Could you check a few things on this drawing? It's one solid part, dimensions in mm from its lowest x, y, z. Round coordinates to 2 decimals unless told otherwise and drop trailing zeros. Write each loop counter-clockwise with the first axis right and the second up, starting at its lowest first coordinate (ties: lowest second). Pieces come first, ordered by that corner, then holes. Notation, with made-up numbers: M 22,18.5 L 57,18.5 A27 ccw 57,50.5 Z; hole C 75.5,41 d4. An arc over 180 degrees is marked long. One line per question, with ' | ' between items. Start each with the question number.
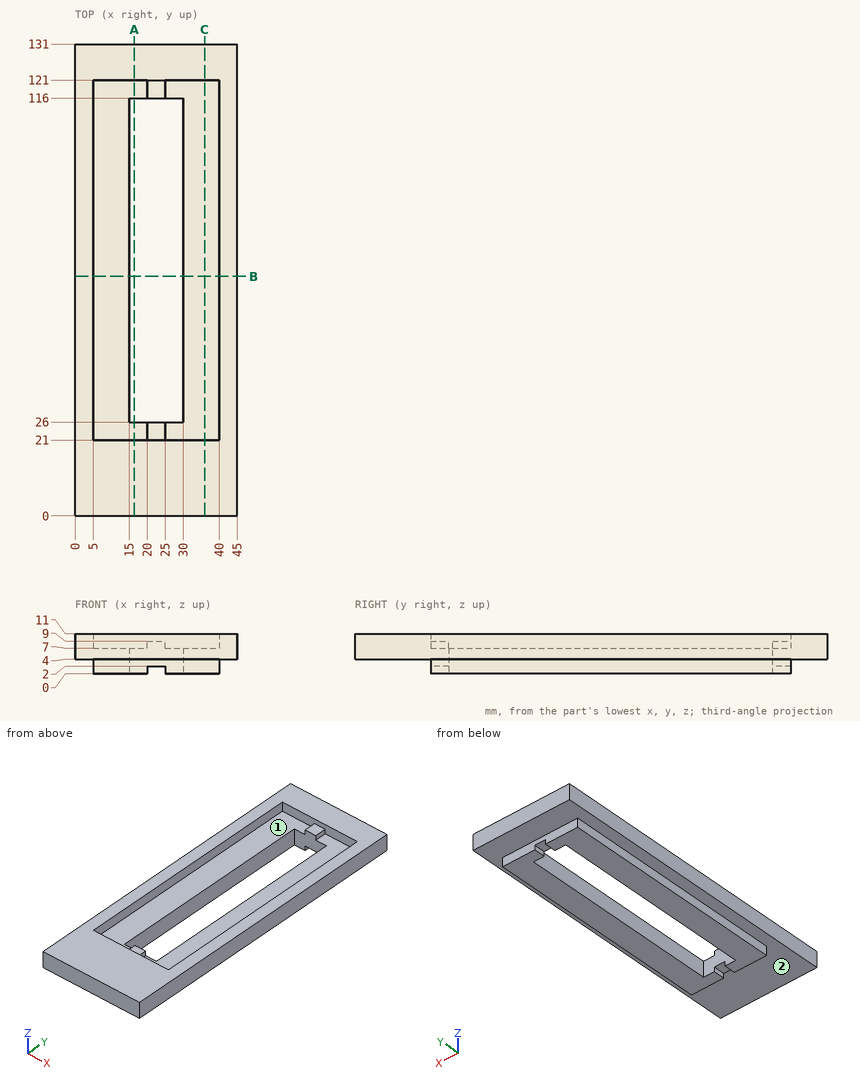
1. Suppose I cut it at C-C (x = 36). Write out the boundary of the cut face in (y, z), and give its area (3 significant figures).
2. I need wall thicknesses on line 1 along Y through (x, z) = (19.5, 1.75); line 2 along X through (y, z) = (95.5, 9.25); line 3 along X through (y, z) = (62, 3.25). Which ranges of each line are inside material? Lowest first, please. Write a range as from..to.
3. Suppose I cut it at A-A (x = 16.5). Write out the boundary of the cut face in (y, z).
4. Suppose I cut it at B-B (y = 66.5). Write out the boundary of the cut face in (x, z), and give its area (3 significant figures).
5. I'm going to push flat-ended pins straight in: P1, Ø7.5, axis at x = 11.5, y = 54, coming from the +Z side; P2, Ø0.6, axis at y = 23, z = 1, coming from the +X side; P3, Ø1, axis at y = 23.5, z = 0.5, coming from the -X side. Where does each tip first touch, or does it pass through?
6. If we mould it in two halves opening along Y, with no side actions, what happens to the marked faces 1 and 2? For each: released by +Y, released by -Y, zero draft, split by the parting line, or undercut.
Computed:
1) outline: M 0,4 L 21,4 L 21,0 L 121,0 L 121,4 L 131,4 L 131,11 L 121,11 L 121,7 L 21,7 L 21,11 L 0,11 Z | area: 917 mm²
2) line 1: y = 21..26, 116..121 | line 2: x = 0..5, 40..45 | line 3: x = 5..15, 30..40
3) outline: M 0,4 L 21,4 L 21,0 L 26,0 L 26,7 L 21,7 L 21,11 L 0,11 Z; M 116,0 L 121,0 L 121,4 L 131,4 L 131,11 L 121,11 L 121,7 L 116,7 Z
4) outline: M 0,4 L 5,4 L 5,0 L 15,0 L 15,7 L 5,7 L 5,11 L 0,11 Z; M 30,0 L 40,0 L 40,4 L 45,4 L 45,11 L 40,11 L 40,7 L 30,7 Z | area: 210 mm²
5) P1: stops at z = 7 | P2: stops at x = 40 | P3: stops at x = 5
6) face 1: undercut | face 2: zero draft
